Source: CAD feature listing. Evaluate the final solid. Frame: model axes, mm. A direction names the side the tool comes from. Coordinates: 2 decimals unless noted, no trailing zeros. Order: outer loops, then holes, each group sorted by start corner. A loop starts at its lowest first (then second) coordinate and runs counter-clockwise, first axis right, second up.
```python
from build123d import *

# Parameters (mm, degrees)
CIRPATTERN1_COUNT = 6


with BuildPart() as part:
    # Sketch1 → Revolve1 (revolve)
    with BuildSketch(Plane.XY, mode=Mode.PRIVATE) as revolve1_sk:
        Polygon((15.5, 21), (0, 21), (0, 26), (38.2, 26), (38.2, 10.5), (34.2, 10.5), (34.2, 15), (26.2, 15), (26.2, 16), (19.2, 16), (19.2, 20), (15.5, 20), align=None)
    revolve(revolve1_sk.sketch.rotate(Axis((-4.437766072, 0, 0), (1, 0, 0)), 90), axis=Axis((-4.437766072, 0, 0), (1, 0, 0)))

    # Sketch3 → M3 Tapped Hole1 (revolve, cut)
    with BuildSketch(Plane(origin=(0, 20.351596989, 11.75), x_dir=(0, 0, 1), z_dir=(0, 1, 0))):
        Polygon((0, 0), (0, 8.251075774), (1.25, 7.5), (1.25, 0), align=None)
    m3_tapped_hole1 = revolve(axis=Axis((-6.35, 20.351596989, 11.75), (1, 0, 0)), mode=Mode.SUBTRACT)

    # CirPattern1: M3 Tapped Hole1 ×6 about axis
    cirpattern1_axis = Axis((0, 0, 0), (1, 0, 0))
    for i in range(1, CIRPATTERN1_COUNT):
        add(m3_tapped_hole1.rotate(cirpattern1_axis, i * 360 / CIRPATTERN1_COUNT), mode=Mode.SUBTRACT)


solid = part.part
```
Q1. Section query C-C on z = 8. Output: boundary loops of the cut face in (x, y), plus the area to 3 significant figures.
Solutions:
outline: (0, -24.74) - (38.2, -24.74) - (38.2, -6.8) - (34.2, -6.8) - (34.2, -12.69) - (26.2, -12.69) - (26.2, -13.86) - (19.2, -13.86) - (19.2, -18.33) - (15.5, -18.33) - (15.5, -19.42) - (0, -19.42) - close; (0, 19.42) - (15.5, 19.42) - (15.5, 18.33) - (19.2, 18.33) - (19.2, 13.86) - (26.2, 13.86) - (26.2, 12.69) - (34.2, 12.69) - (34.2, 6.8) - (38.2, 6.8) - (38.2, 24.74) - (0, 24.74) - close
area: 701 mm2
Q2. Material intervals for line 1 along Y through (x, z) = (4.25, -11.75); line 2 along X through (y, z) = (-20.5, -1.5); line 3 along Z through (x, y) = (8, -1), sorted ascending.
Solutions:
line 1: y = -23.19 to -21.6, -19.1 to -17.41, 17.41 to 19.1, 21.6 to 23.19
line 2: x = 15.5 to 38.2
line 3: z = -25.98 to -20.98, 20.98 to 25.98
Q3. Section query D-D on y = -12. Output: boundary loops of the cut face in (x, z), plus the area to 3 significant figures.
Solutions:
outline: (0, -23.07) - (38.2, -23.07) - (38.2, 23.07) - (0, 23.07) - (0, 17.23) - (15.5, 17.23) - (15.5, 16) - (19.2, 16) - (19.2, 10.58) - (26.2, 10.58) - (26.2, 9) - (34.2, 9) - (34.2, -9) - (26.2, -9) - (26.2, -10.58) - (19.2, -10.58) - (19.2, -16) - (15.5, -16) - (15.5, -17.23) - (0, -17.23) - close
area: 817 mm2
Q4. Set-up query: faces 1 (the cylindrical face through (3.698, -19.507, -10.829)), 2 (the flat face through (0, 21.1, 2)). Return all of +Z, -Z, +X, -X, +Y, -Y with unobstructed straight access to the full face (end or side cutting, diameter ignored); none if empty.
Solutions:
face 1: -X
face 2: +Z, -Z, -X, +Y, -Y
Q5. Pin query (flat end, axial travel): P1, Ø12, axis at y = 2.5, z = 3.5, coming from the -X side; P2, Ø10, axis at x = 26.5, z = 16, coming from the -Y side; P3, Ø8, axis at x = 27.5, y = -3.5, coming from the +Z side; P4, Ø3, axis at x = 18.5, z = -13.5, coming from the +Y side. Return the tip coordinate at first contact, or that it passes through.
Solutions:
P1: passes through
P2: stops at y = -23.56
P3: stops at z = 26
P4: stops at y = 23.07
Q6. Section query B-B on x = 10. Output: boundary loops of the cut face in (y, z).
Solutions:
outline: circle Ø52 at (0, 0); hole circle Ø42 at (0, 0)
Q7. Pull-direction query (Z, two-part tool) for faces 3 (the flat face through (15.5, 8, -19)), 4 (the flat face through (38.2, 0, 11)); classes: pulls with the +Z half, pulls with the -Z half, needs draft (parallel to the pull), parting line crosses it, or undercut.
Solutions:
face 3: undercut
face 4: needs draft
Q8. Section query A-A on y = 6.5. Output: boundary loops of the cut face in (x, z), plus the area to 3 significant figures.
Solutions:
outline: (0, -25.17) - (38.2, -25.17) - (38.2, -8.25) - (34.2, -8.25) - (34.2, -13.52) - (26.2, -13.52) - (26.2, -14.62) - (19.2, -14.62) - (19.2, -18.91) - (15.5, -18.91) - (15.5, -19.97) - (0, -19.97) - close; (0, 19.97) - (15.5, 19.97) - (15.5, 18.91) - (19.2, 18.91) - (19.2, 14.62) - (26.2, 14.62) - (26.2, 13.52) - (34.2, 13.52) - (34.2, 8.25) - (38.2, 8.25) - (38.2, 25.17) - (0, 25.17) - close
area: 677 mm2
